Check sheet for the drawn part. Datum: minimum x, y, z corner. Units: mm. A direction names the side the tool comes from. Coordinates: 2 decimals unless noted, no trailing zeros. Loops run counter-clockwise (first coordinate to the right, second up) from the corner with the lowest first, then second, coordinate; pieces in that order, holes last. Notation, with made-up numbers: (65, -10) - (73, -10) arc R4 ccw to (73, -5) - close; hole circle Ø3 at (-39, -4). An arc over 180 degrees is marked (long way). Answer as CSV lines item,"result". Start each with the question number.
1. Cross-section at C-C (y = 8). Enter the section's corners in (x, z) (3 decimals).
2. Cross-section at B-B (x = 17). Enter the section's corners in (y, z) (3 decimals), plus the area to 3 significant figures.
3. Cross-section at D-D (z = 26). Enter the section's corners in (x, y) (3 decimals).
4. Cross-section at A-A (z = 2). Enter the section's corners in (x, y) (3 decimals).
5. Release check for a two-part mould opening along Z. For the marked faces 3 and 4 record: pulls with the +Z half, pulls with the -Z half, needs draft (parallel to the pull), parting line crosses it, or undercut.
6. Set-up check for the marked faces 1 and 2: record each of +Z, -Z, +X, -X, +Y, -Y from which the full face is reachable in a straight line by a thin tool's end or side.
7. Gauge pin test, flat ends, axial feed: P1, Ø4, axis at y = 3.5, z = 11, coming from the -X side; P2, Ø5, axis at x = 26.035, z = 22.225, coming from the -Y side (3 decimals); P3, Ø2, axis at x = 14.5, y = 1, coming from the -Z side; P4, Ø5, axis at x = 28, y = 7, coming from the +Z side. Record the tip position at first contact, or that the pin passes through.
8. Material ranges on line 1 (Z direction, x = 6.5, y = 8.5); line 2 (Y direction, x = 9.5, z = 18.5) (3 decimals); line 3 (X direction, y = 7.75, z = 9), recorded low to high. Write a range as [from, to].
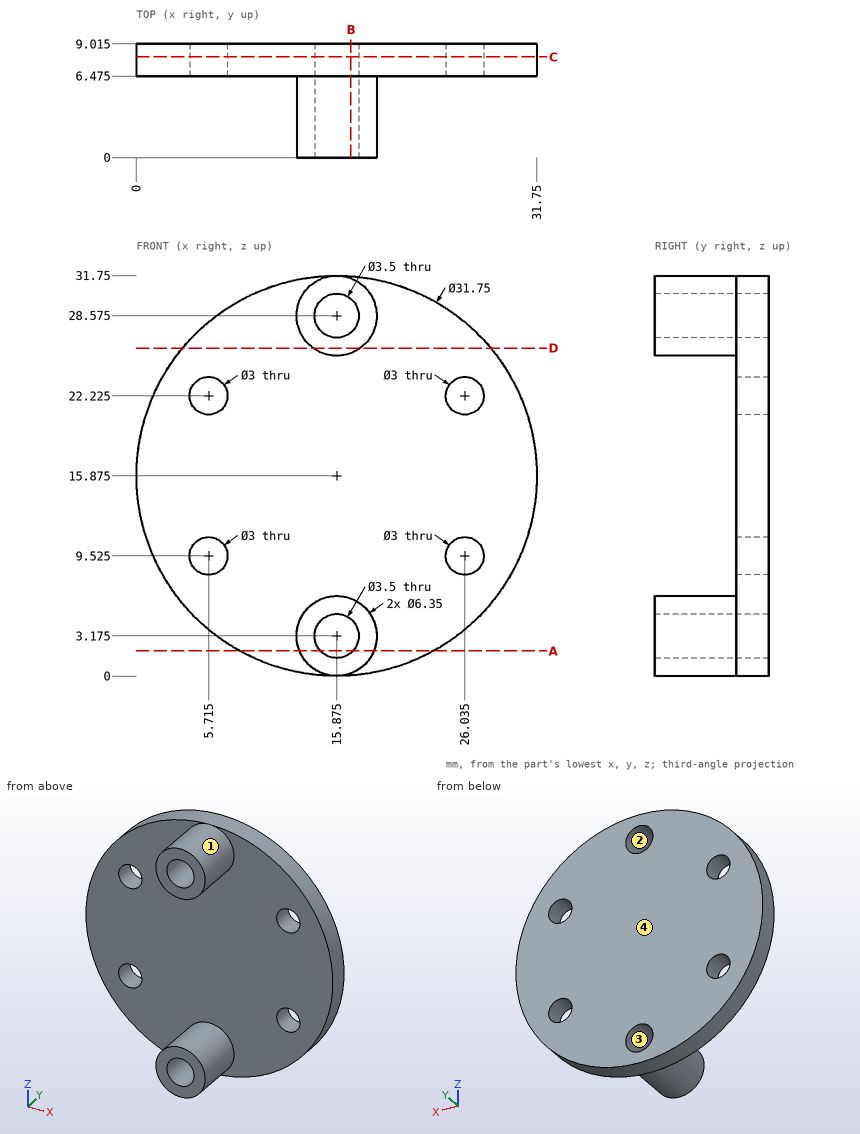
Values follow:
1,outline,"circle Ø31.75 at (15.875, 15.875); hole circle Ø3 at (5.715, 9.525); hole circle Ø3 at (5.715, 22.225); hole circle Ø3.5 at (15.875, 3.175); hole circle Ø3.5 at (15.875, 28.575); hole circle Ø3 at (26.035, 9.525); hole circle Ø3 at (26.035, 22.225)"
2,outline,"(0, 0.206) - (6.475, 0.206) - (6.475, 0.04) - (9.015, 0.04) - (9.015, 1.835) - (0, 1.835) - close; (0, 4.515) - (9.015, 4.515) - (9.015, 27.235) - (0, 27.235) - (0, 25.606) - (6.475, 25.606) - (6.475, 6.144) - (0, 6.144) - close; (0, 29.915) - (9.015, 29.915) - (9.015, 31.71) - (6.475, 31.71) - (6.475, 31.544) - (0, 31.544) - close"
2,area,"109 mm²"
3,outline,"(3.648, 6.475) - (14.018, 6.475) - (14.018, 0) - (17.732, 0) - (17.732, 6.475) - (28.102, 6.475) - (28.102, 9.015) - (3.648, 9.015) - close"
4,outline,"(8.161, 6.475) - (12.925, 6.475) - (12.925, 0) - (14.578, 0) - (14.578, 9.015) - (8.161, 9.015) - close; (17.172, 0) - (18.825, 0) - (18.825, 6.475) - (23.589, 6.475) - (23.589, 9.015) - (17.172, 9.015) - close"
5,face 3,"undercut"
5,face 4,"needs draft"
6,face 1,"-Y"
6,face 2,"+Y, -Y"
7,P1,"passes through"
7,P2,"stops at y = 6.475"
7,P3,"stops at z = 0.02"
7,P4,"stops at z = 28.5"
8,line 1,"z = [3.06, 8.25], [10.8, 20.95], [23.5, 28.69]"
8,line 2,"y = [6.475, 9.015]"
8,line 3,"x = [1.57, 4.31], [7.12, 24.63], [27.44, 30.18]"
